```python
from build123d import *

# Parameters (mm, degrees)
F1_DEPTH    = 15
F2_T1_DEPTH = 28.8982001462
F2_T3_DEPTH = 16.0188013663
F3_T1_DEPTH = 30.3272306083
F4_R        = 1.5


# Not quite as in the source:
# - a fillet or chamfer that OpenCascade refuses, or shapes differently, is made with other operations: its cross-section is extruded or revolved along the edge and cut away or added
# - a feature names something its author has since deleted; it is built from what else it names


with BuildPart() as f1:
    # F0 (on Front) → F1 (new body)
    with BuildSketch(Plane.XZ):
        with BuildLine():
            ThreePointArc((64.5076036134, -1.44), (63.120788421, -0.0985070956), (61.9563763345, 1.44))
            Line((61.9563763345, 1.44), (-72.5, 1.44))
            Line((-72.5, 1.44), (-72.5, -1.44))
            Line((-72.5, -1.44), (64.5076036134, -1.44))
        make_face()
        with BuildLine():
            Line((61.9563763345, 1.44), (65.6232565847, 1.44))
            ThreePointArc((65.6232565847, 1.44), (63.599073082, 11.9377338961), (72.5, 17.86))
            Line((72.5, 17.86), (72.5, 20.74))
            ThreePointArc((72.5, 20.74), (61.5038870504, 14.2171956852), (61.9563763345, 1.44))
        make_face()
        with BuildLine():
            ThreePointArc((72.5, -1.44), (68.7722661039, -0.690926918), (65.6232565847, 1.44))
            Line((65.6232565847, 1.44), (61.9563763345, 1.44))
            ThreePointArc((61.9563763345, 1.44), (63.120788421, -0.0985070956), (64.5076036134, -1.44))
            Line((64.5076036134, -1.44), (72.5, -1.44))
        make_face()
    extrude(amount=F1_DEPTH)

    # F2: chamfer of 0.2 on 2 edges, made by hand

    # F2_s2 → F2_t1 (cut)
    with BuildSketch(Plane.XZ.offset(-6.9491000731)):
        with BuildLine():
            Line((69.7215112021, -1.44), (69.7779272183, -1.0481218274))
            ThreePointArc((69.7779272183, -1.0481218274), (71.1249319352, -1.3415280357), (72.5, -1.44))
            Line((72.5, -1.44), (69.7215112021, -1.44))
        make_face()
    extrude(amount=F2_T1_DEPTH, mode=Mode.SUBTRACT)

    # F2_s4 → F2_t3 (cut)
    with BuildSketch(Plane.XZ.offset(-0.5094006831)):
        with BuildLine():
            Line((72.3040609137, 17.8580105656), (72.5, 18.0579693338))
            Line((72.5, 18.0579693338), (72.5, 17.86))
            ThreePointArc((72.5, 17.86), (72.399196155, 17.8594734874), (72.3040609137, 17.8580105656))
        make_face()
    extrude(amount=F2_T3_DEPTH, mode=Mode.SUBTRACT)

    # F3: chamfer of 2.98 on 1 edges, made by hand

    # F3_s2 → F3_t1 (cut)
    with BuildSketch(Plane.XZ.offset(-7.6636153041)):
        Polygon((-72.5, -1.54), (-69.52, 1.44), (-72.5, 1.44), align=None)
    extrude(amount=F3_T1_DEPTH, mode=Mode.SUBTRACT)

    # F4
    f4_edges = [f1.edges().sort_by_distance(p)[0] for p in [
        (72.5, -7.5, 20.74),
    ]]
    fillet(f4_edges, radius=F4_R)


solid = f1.part
```
Geometry: final body of the model. Coordinates: model frame, mm. Round coordinates to 2 decimals unless told otherwise and drop trailing zeros. Order: outer loops, then holes, each group sorted by start corner. A loop starts at its lowest first (then second) coordinate and runs counter-clockwise, first axis right, second up. Notation, with made-up numbers: (53, 61.5) - (92, 61.5) arc R21 ccw to (92, 72.5) - close; hole circle Ø9 at (11, 75.25). An arc over 180 degrees is marked (long way). Write item = value, one per line. Start each with the question number.
Q1. Pull-direction query (Z, two-part tool) for faces 1 (the flat face through (-2, -7, -1.44)), 2 (the flat face through (5, -15, 1)), 3 (the cylindrical face through (61.195, -7.395, 13.613)); classes: +Z half, -Z half, draft (parallel to the pull), parting line (faces both ways), or undercut.
Q2. Cut plane C-C on z = 12.25. Return the cut outline in (x, y).
Q3. Pin query (flat end, axial travel): pin 1 (5 mm diameter, centred on x = -45, z = 6, fed in from -Y); pin 2 (4.5 mm diameter, centred on x = -22, y = -7.5, fed in from +Z); pin 3 (3 mm diameter, centred on y = -8.5, z = 13.5, fed in from -X); pin 4 (1.5 mm diameter, centred on y = -8, z = 9, fed in from -X). Return the tip coordinate at first contact, or that it passes through.
Q4. Cut plane B-B on x = 27. Return the cut outline in (y, z).
Q5. Ray query, line 1 (Z direction, x = 12.5, y = -8.5); line 2 (X direction, y = -3.75, z = 0); line 3 (X direction, y = -12, z = 12.25). Return the intervals inside material, ascending. Write a range as from..to.
Q6. Cut plane A-A on y = -11.25. Return the cut outline in (x, z), and give its area (3 significant figures).
Outcome:
q1.face_1 = -Z half
q1.face_2 = draft
q1.face_3 = undercut
q2.outline = (60.64, -15) - (63.74, -15) - (63.74, 0) - (60.64, 0) - close
q3.pin_1 = through
q3.pin_2 = 1.44
q3.pin_3 = 60.56
q3.pin_4 = 59.97
q4.outline = (-15, -1.44) - (0, -1.44) - (0, 1.44) - (-15, 1.44) - close
q5.line_1 = -1.44..1.44
q5.line_2 = -70.96..67.43
q5.line_3 = 60.64..63.74
q6.outline = (-72.4, -1.44) - (69.72, -1.44) - (69.78, -1.05) arc R9.65 cw to (72.3, 17.86) - (72.5, 18.06) - (72.5, 19.14) arc R1.5 ccw to (70.8, 20.62) arc R12.53 ccw to (61.96, 1.44) - (-69.52, 1.44) - close
q6.area = 470 mm^2
